Source: three-view drawing plus pictorial views. Frame: mm from the lowest corner of the part. A direction names the side the tool comes from. Coordinates: 2 decimals unless noted, no trailing zeros. Write each loop counter-clockwise with the first axis right and the second up, starting at its lowest first coordinate (ties: lowest second). Pieces come first, ordered by that corner, then holes. Notation, with made-up numbers: M 80,35.25 L 84,35.25 A22 cw 84,70.25 Z; hole C 73.5,73 d11. An arc over 180 degrees is marked long. Use CSV: the item, a comma, the result in double quotes.
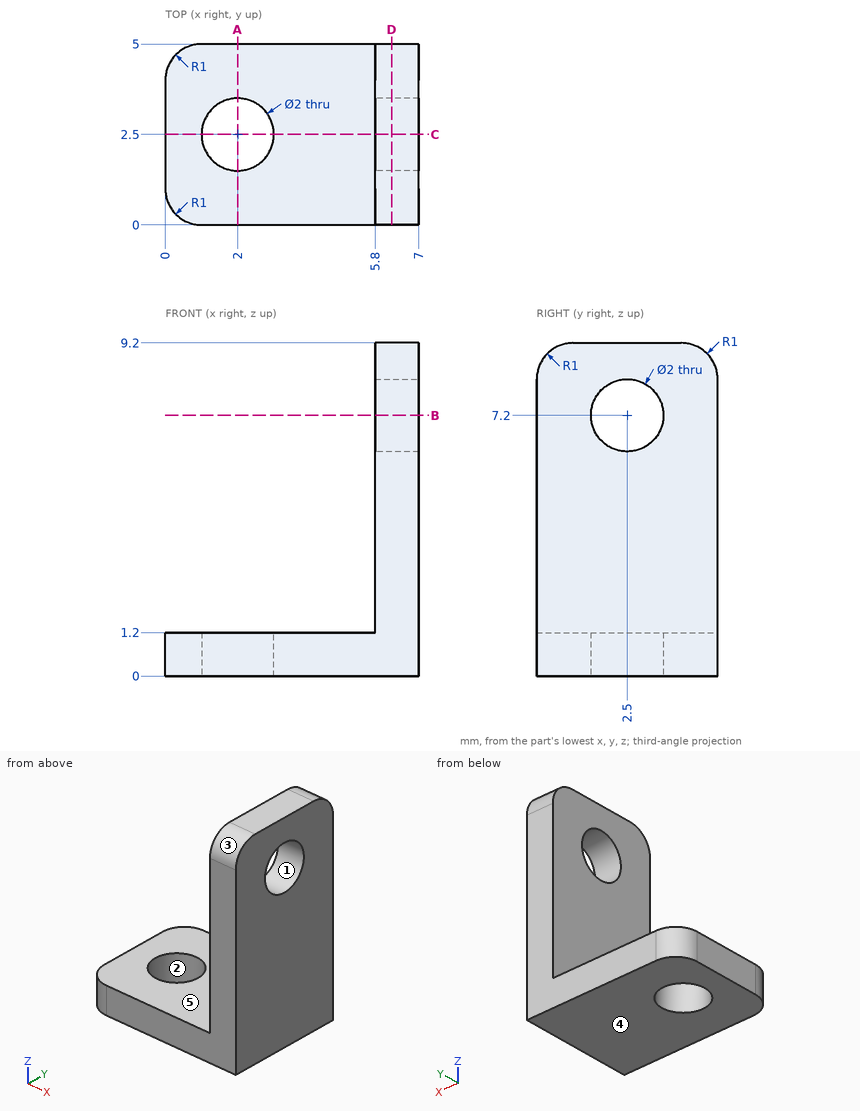
1. Material intervals for line 1 (Y direction, x = 2, z = 0.7); line 2 (Z direction, x = 5.5, y = 4.6); line 3 (X direction, y = 1.5, z = 5), sorted ascending. Write a range as [from, to].
Resolved:
line 1,"y = [0, 1.5], [3.5, 5]"
line 2,"z = [0, 1.2]"
line 3,"x = [5.8, 7]"
2. Section B-B (z = 7.2). Return loops of the section in (x, y), then the cut area to 3 significant figures.
Resolved:
outline,"M 5.8,0 L 7,0 L 7,1.5 L 5.8,1.5 Z; M 5.8,3.5 L 7,3.5 L 7,5 L 5.8,5 Z"
area,"3.60 mm^2"
3. Mould query, pull axis Z, two halves, no side actions, for the marked faces 1, 2 and 3. Classes: pulls with the +Z half, pulls with the -Z half, needs draft (parallel to the pull), parting line crosses it, or undercut.
Resolved:
face 1,"undercut"
face 2,"needs draft"
face 3,"pulls with the +Z half"
4. Section A-A (x = 2). Return loops of the section in (y, z).
Resolved:
outline,"M 0,0 L 1.5,0 L 1.5,1.2 L 0,1.2 Z; M 3.5,0 L 5,0 L 5,1.2 L 3.5,1.2 Z"
5. Section D-D (x = 6.25). Return loops of the section in (y, z), then the cut area to 3 significant figures.
Resolved:
outline,"M 0,0 L 5,0 L 5,8.2 A1 ccw 4,9.2 L 1,9.2 A1 ccw 0,8.2 Z; hole C 2.5,7.2 d2"
area,"42.4 mm^2"
6. Contact query for flat-ended pins moving along their axis: pin 1 Ø2.5 at (x, y) = (2, 2.5) entering from +Z; pin 2 Ø1.6 at (y, z) = (2.5, 7.2) entering from +X; pin 3 Ø3 at (y, z) = (1, 5.5) entering from -X. Output: stop coordinate, or through.
Resolved:
pin 1,"stops at z = 1.2"
pin 2,"passes through"
pin 3,"stops at x = 5.8"
7. Section C-C (y = 2.5). Return loops of the section in (x, z), then the cut area to 3 significant figures.
Resolved:
outline,"M 0,0 L 1,0 L 1,1.2 L 0,1.2 Z; M 3,0 L 7,0 L 7,6.2 L 5.8,6.2 L 5.8,1.2 L 3,1.2 Z; M 5.8,8.2 L 7,8.2 L 7,9.2 L 5.8,9.2 Z"
area,"13.2 mm^2"
8. Access query for the marked faces 4 and 5. Directions: +Z, -Z, +X, -X, +Y, -Y. A direction counts if a zero-diameter tool reaches every point of the face in a straight line with its end or side. Return the directions, or none.
Resolved:
face 4,"-Z, +X, -X, +Y, -Y"
face 5,"+Z, -X, +Y, -Y"
